Can you work these out from the model? Positions are in its coordinate system, mm. Round coordinates to 2 decimals unless told otherwise and drop trailing zeros. Loops run counter-clockwise (first coordinate to the right, second up) from the corner with the lowest first, then second, coordinate; pieces in that order, holes last.
(1) If I drill on line 1 along X through (y, z) = (1.8, -75); line 2 along Z through (x, y) = (75, 1.9); line 3 along Z through (x, y) = (77, 2.45), over which ranges is the centre line in solid material (lowest first)?
(2) I want a section at A-A on x = 75. Write out the boundary of the cut face in (y, z), plus the area to 3 significant figures.
(3) I want a section at C-C on x = 101. Write out the boundary of the cut face in (y, z).
(4) I want a section at B-B on z = -75. Write out the boundary of the cut face in (x, y).
(5) Will these pins go through, and if not, where does the flat tip stop? pin 1 Ø6 at (x, z) = (40.5, -89) entering from -Y; pin 2 Ø1.5 at (x, y) = (113, 2.5) entering from +Z; pin 3 Ø1.5 at (y, z) = (1, -16) entering from +X.
from build123d import *

# Parameters (mm, degrees)
SKETCH1_R           = 2.5
BOSS_EXTRUDE1_DEPTH = 3


with BuildPart() as part:
    # Sketch1 → Boss-Extrude1 (new body)
    with BuildSketch(Plane(origin=(0, 0, 0), x_dir=(1, 0, 0), z_dir=(0, 1, 0))):
        Polygon((59.9, 0), (90.1, 0), (90.1, 3), (119.9, 3), (119.9, 0), (150, 0), (150, 10.1), (147, 10.1), (147, 29.9), (150, 29.9), (150, 150), (0, 150), (0, 29.9), (3, 29.9), (3, 10.1), (0, 10.1), (0, 0), (30.1, 0), (30.1, 3), (59.9, 3), align=None)
        with Locations((75, 75)):
            Circle(SKETCH1_R, mode=Mode.SUBTRACT)
    extrude(amount=BOSS_EXTRUDE1_DEPTH)


solid = part.part
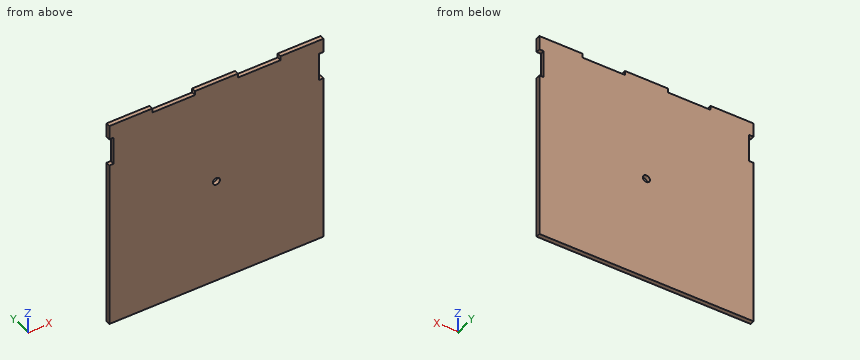
Filled sheet:
1. line 1: x = 0 to 72.5, 77.5 to 150
1. line 2: z = -150 to -77.5, -72.5 to 0
1. line 3: z = -150 to -76.5, -73.5 to 0
2. outline: (0, -150) - (3, -150) - (3, -77.5) - (0, -77.5) - close; (0, -72.5) - (3, -72.5) - (3, 0) - (0, 0) - close
2. area: 435 mm2
3. outline: (0, -150) - (3, -150) - (3, -3) - (0, -3) - close
4. outline: (0, 0) - (72.5, 0) - (72.5, 3) - (0, 3) - close; (77.5, 0) - (150, 0) - (150, 3) - (77.5, 3) - close
5. pin 1: stops at y = 0
5. pin 2: stops at z = -3
5. pin 3: stops at x = 147
